Build history of the part. All positions in model axes, mm. Face numbers are marked on the shaded views. Round coordinates to 2 decimals unless told otherwise and drop trailing zeros. Write each loop counter-clockwise with the first axis right and the second up, starting at its lowest first coordinate (ties: lowest second). Pieces come first, ordered by that corner, then holes.
Item 1: Wall check: probe 1 along Z at (x, y) = (-0.75, 4.5); probe 2 along Z at (x, y) = (-6.75, 1.5); probe 3 along X at (y, z) = (10.75, -5). Give the ranges that are in metal, low to high.
Item 2: Mould opens along Z. For the marked faces 1, 2 and 3 say: +Z half, -Z half, draft (parallel to the pull), parting line (faces both ways), or undercut.
Item 3: Drop flat-ended pins along their axis: pin 1 Ø10 at (x, z) = (5, 1) entering from -Y; pin 2 Ø6 at (x, y) = (-9, 6) entering from -Z; pin 3 Ø5 at (x, y) = (9, 1.5) entering from +Z. Give the stop position or say it passes through.
Item 4: Band-saw the part on B-B, the plane y = 4.25. Write the cut outline in (x, z).
Item 5: Band-saw the part on A-A, the plane y = 5.75. Write the cut outline in (x, z).
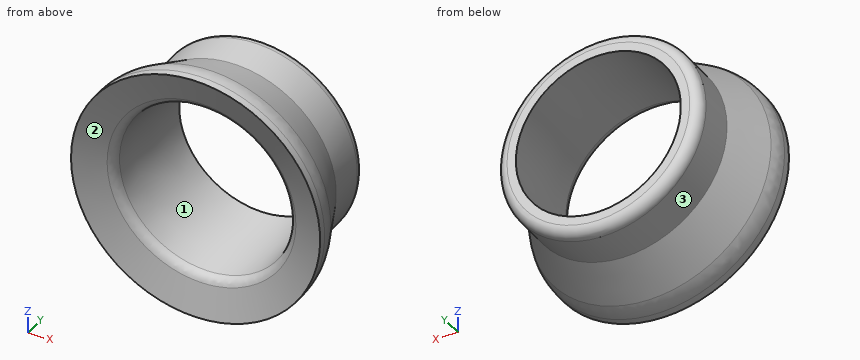
```python
from build123d import *

# Parameters (mm, degrees)
FILLET1_R = 1
FILLET2_R = 1
FILLET3_R = 4


with BuildPart() as part:
    # Sketch2 → Revolve1 (revolve)
    with BuildSketch(Plane.XY, mode=Mode.PRIVATE) as revolve1_sk:
        Polygon((0, 0), (12, 0), (12, 1.6), (9.8, 6.5), (9.8, 11), (0, 11), align=None)
    revolve(revolve1_sk.sketch.rotate(Axis((0, 11, 0), (0, -1, 0)), 180), axis=Axis((0, 11, 0), (0, -1, 0)))

    # Sketch4 → Cut-Revolve1 (revolve, cut)
    with BuildSketch(Plane.XY, mode=Mode.PRIVATE) as cut_revolve1_sk:
        Polygon((0, 0), (0, 11), (7.95, 11), (8.45, 1.2), (12, 0), align=None)
    revolve(cut_revolve1_sk.sketch.rotate(Axis((0, 0, 0), (0, 1, 0)), 90), axis=Axis((0, 0, 0), (0, 1, 0)), mode=Mode.SUBTRACT)

    # Fillet1
    fillet1_edges = [part.edges().sort_by_distance(p)[0] for p in [
        (9.8, 11, 0),
    ]]
    fillet(fillet1_edges, radius=FILLET1_R)

    # Fillet2
    fillet2_edges = [part.edges().sort_by_distance(p)[0] for p in [
        (0, 1.2, 8.45),
    ]]
    fillet(fillet2_edges, radius=FILLET2_R)

    # Fillet3
    fillet3_edges = [part.edges().sort_by_distance(p)[0] for p in [
        (12, 1.6, 0),
    ]]
    fillet(fillet3_edges, radius=FILLET3_R)


solid = part.part
```
Results:
1. probe 1: z = -10.67 to -8.25, 8.25 to 10.67
1. probe 2: z = -9.83 to -5.18, 5.18 to 9.83
1. probe 3: x = -8.03 to -6.2, 6.2 to 8.03
2. face 1: undercut
2. face 2: undercut
2. face 3: parting line
3. pin 1: stops at y = 0.64
3. pin 2: stops at z = -8.59
3. pin 3: stops at z = 10.05
4. outline: circle Ø21.62 at (0, 0); hole circle Ø16.59 at (0, 0)
5. outline: circle Ø20.27 at (0, 0); hole circle Ø16.44 at (0, 0)
